```python
from build123d import *

# Parameters (mm, degrees)
BOSS_EXTRUDE1_DEPTH = 45
BOSS_EXTRUDE2_DEPTH = 5
SKETCH4_W           = 5
SKETCH4_H           = 5
SKETCH4_H_2         = 15
SKETCH4_W_2         = 13.596951961
CUT_EXTRUDE2_DEPTH  = 45
SKETCH5_R           = 5
CUT_EXTRUDE3_DEPTH  = 45
SKETCH6_R           = 1
CUT_EXTRUDE4_DEPTH  = 10
BOSS_EXTRUDE3_DEPTH = 5
SKETCH9_R           = 1.5
CUT_EXTRUDE5_DEPTH  = 5


with BuildPart() as part:
    # Sketch1 → Boss-Extrude1 (new body)
    with BuildSketch(Plane(origin=(0, 0, 0), x_dir=(1, 0, 0), z_dir=(0, 1, 0))):
        Polygon((-62, 72), (62, 72), (62, 62), (72, 62), (72, -62), (62, -62), (62, -72), (-62, -72), (-62, -62), (-72, -62), (-72, 62), (-62, 62), align=None)
        Polygon((-62, 52), (-62, -52), (-52, -52), (-52, -62), (52, -62), (52, -52), (62, -52), (62, 52), (52, 52), (52, 62), (-52, 62), (-52, 52), align=None, mode=Mode.SUBTRACT)
    extrude(amount=BOSS_EXTRUDE1_DEPTH)

    # Sketch2 → Boss-Extrude2 (add)
    with BuildSketch(Plane(origin=(0, 45, 0), x_dir=(1, 0, 0), z_dir=(0, 1, 0))):
        Polygon((-62, 72), (62, 72), (62, 62), (72, 62), (72, -62), (62, -62), (62, -72), (-62, -72), (-62, -62), (-72, -62), (-72, 62), (-62, 62), align=None)
    extrude(amount=BOSS_EXTRUDE2_DEPTH)

    # Sketch4 → Cut-Extrude2 (cut)
    with BuildSketch(Plane.XZ):
        with Locations((54.5, 54.5)):
            Rectangle(SKETCH4_W, SKETCH4_H)
        with Locations((-64.5, 7.5)):
            Rectangle(SKETCH4_W, SKETCH4_H_2)
        with Locations((58.798475981, -54.5)):
            Rectangle(SKETCH4_W_2, SKETCH4_H)
    extrude(amount=-CUT_EXTRUDE2_DEPTH, mode=Mode.SUBTRACT)

    # Sketch5 → Cut-Extrude3 (cut)
    with BuildSketch(Plane.XZ):
        with Locations((11.02, -60.75)):
            Circle(SKETCH5_R)
    extrude(amount=-CUT_EXTRUDE3_DEPTH, mode=Mode.SUBTRACT)

    # Sketch6 → Cut-Extrude4 (cut)
    with BuildSketch(Plane.XZ):
        with Locations(Location((0, 66.667049072, 0), (0, 0, 270))):
            Circle(SKETCH6_R)
        with Locations(Location((0, -66.67, 0), (0, 0, 270))):
            Circle(SKETCH6_R)
    extrude(amount=-CUT_EXTRUDE4_DEPTH, mode=Mode.SUBTRACT)

    # Sketch8 → Boss-Extrude3 (add)
    with BuildSketch(Plane(origin=(0, 0, 0), x_dir=(-1, 0, 0), z_dir=(0, -1, 0))):
        with BuildLine():
            Line((62, 72), (62, 62))
            Line((62, 62), (72, 62))
            ThreePointArc((72, 62), (69.071067812, 69.071067812), (62, 72))
        make_face()
        with BuildLine():
            Line((62, -72), (62, -62))
            Line((62, -62), (72, -62))
            ThreePointArc((72, -62), (69.071067812, -69.071067812), (62, -72))
        make_face()
        with BuildLine():
            Line((-62, -62), (-72, -62))
            ThreePointArc((-72, -62), (-69.071067812, -69.071067812), (-62, -72))
            Line((-62, -72), (-62, -62))
        make_face()
        with BuildLine():
            Line((-62, 62), (-72, 62))
            ThreePointArc((-72, 62), (-69.071067812, 69.071067812), (-62, 72))
            Line((-62, 72), (-62, 62))
        make_face()
    extrude(amount=-BOSS_EXTRUDE3_DEPTH)

    # Sketch9 → Cut-Extrude5 (cut)
    with BuildSketch(Plane(origin=(0, 5, 0), x_dir=(1, 0, 0), z_dir=(0, 1, 0))):
        with Locations(Location((-67, -67, 0), (0, 0, 270))):
            Circle(SKETCH9_R)
        with Locations(Location((67, -67, 0), (0, 0, 90))):
            Circle(SKETCH9_R)
        with Locations(Location((67, 67, 0), (0, 0, 270))):
            Circle(SKETCH9_R)
        with Locations(Location((-67, 67, 0), (0, 0, 90))):
            Circle(SKETCH9_R)
    extrude(amount=-CUT_EXTRUDE5_DEPTH, mode=Mode.SUBTRACT)


solid = part.part
```
Check sheet for the modelled part. Datum: model origin and axes. Units: mm. A direction names the side the tool comes from. Round coordinates to 2 decimals unless told otherwise and drop trailing zeros. Loops run counter-clockwise (first coordinate to the right, second up) from the corner with the lowest first, then second, coordinate; pieces in that order, holes last. Notation, with made-up numbers: (-25, 37) - (21, 37) arc R18 cw to (21, 61) - close; hole circle Ø6 at (-10.75, 9). An arc over 180 degrees is marked (long way). Write item = value, one per line. Start each with the question number.
Q1. Depth check by flat-ended pin: P1, Ø8, axis at x = 68.5, z = 64.5, coming from the +Y side; P2, Ø8, axis at x = 47.5, z = 9.5, coming from the -Y side; P3, Ø3, axis at y = 30, z = 68, coming from the +X side; P4, Ø2.5, axis at x = -65.5, y = 25.5, coming from the +Z side. Enter the tip coordinate at first touch or a pass-through.
Q2. Thickness scan on L1, parallel to Z at x = 28, y = 16; L2, parallel to X at y = 3.4, z = -67. Record the ranges inside material, lowest first.
Q3. Section check D-D (y = 8). Count the separate pieces of the cut face and the enclosed holes in it, plus the area to 3 significant figures.
Q4. Section check B-B (x = -22). Record the boundary of the cut face in (y, z), plus the area to 3 significant figures.
Q5. Section check C-C (z = 9.5). Record the boundary of the cut face in (x, y).
Q6. Release check for a two-part mould opening along Z. For faces 1 (the face through (-62, 27, 67)), 2 (the face through (-69.15, 2.46, -68.99)), 3 (the face through (57, 22, 54)), 4 (the face through (69.15, 2.46, 68.99)) record: pulls with the +Z half, pulls with the -Z half, needs draft (parallel to the pull), parting line crosses it, or undercut.
Q7. Access from +Z, -Z, +X, -X, +Y, -Y to the whole of each face (thin tool, end or side, straight path). Record for faces 5 (the face through (-65, 5, -66)), 6 (the face through (-57, 22, -52)), 7 (the face through (65, 0, -1)).
Derived:
q1.P1 = 50
q1.P2 = 45
q1.P3 = 62
q1.P4 = 62
q2.L1 = -72 to -62, 62 to 72
q2.L2 = -70.66 to -68.5, -65.5 to -0.94, 0.94 to 65.5, 68.5 to 70.66
q3.separate_pieces = 1
q3.enclosed_holes = 3
q3.area = 5,160 mm^2
q4.outline = (0, -72) - (50, -72) - (50, 72) - (0, 72) - (0, 62) - (45, 62) - (45, -62) - (0, -62) - close
q4.area = 1,620 mm^2
q5.outline = (-72, 0) - (-67, 0) - (-67, 45) - (62, 45) - (62, 0) - (72, 0) - (72, 50) - (-72, 50) - close
q6.face_1 = needs draft
q6.face_2 = pulls with the -Z half
q6.face_3 = undercut
q6.face_4 = pulls with the +Z half
q7.face_5 = -Z, -X, +Y
q7.face_6 = -Y
q7.face_7 = +Z, -Z, +X, -X, -Y
